Can you work these out from the model? Positions are in its coordinate system, mm. A direction names the side the tool comes from. Give positions to 0.01 mm unless a question says otherwise; leave off trailing zeros. Write each loop counter-clockwise with the first axis right and the second up, starting at its lowest first coordinate (ties: lowest second). Pieces come first, ordered by that corner, then holes. Notation, with made-up numbers: (-18.5, 3) -> (5.5, 3) arc R18 cw to (5.5, 23) -> close; hole circle Ø3 at (67, 88). An arc over 180 degrees is marked (long way). One line per item, written item: value.
from build123d import *

# Parameters (mm, degrees)
SKETCH1_W           = 40
SKETCH1_H           = 27
BOSS_EXTRUDE1_DEPTH = 30
CUT_EXTRUDE1_DEPTH  = 10
SKETCH3_R           = 2.5
CUT_EXTRUDE2_DEPTH  = 30
CUT_EXTRUDE5_START  = -10.62
CUT_EXTRUDE5_DEPTH  = 9
SKETCH10_W          = 20
SKETCH10_H          = 9
CUT_EXTRUDE7_DEPTH  = 6.8
SKETCH12_W          = 20
SKETCH12_H          = 9
CUT_EXTRUDE10_DEPTH = 6.8
FILLET1_R           = 4
SKETCH15_R          = 4.1
CUT_EXTRUDE12_DEPTH = 4
SKETCH16_R          = 2.5
CUT_EXTRUDE13_DEPTH = 4


with BuildPart() as part:
    # Sketch1 → Boss-Extrude1 (new body)
    with BuildSketch(Plane(origin=(0, 0, 0), x_dir=(1, 0, 0), z_dir=(0, 1, 0))):
        with Locations((-2.846153846, 4.313186813)):
            Rectangle(SKETCH1_W, SKETCH1_H)
    extrude(amount=BOSS_EXTRUDE1_DEPTH)

    # Sketch2 → Cut-Extrude1 (cut)
    with BuildSketch(Plane(origin=(0, 0, -17.813186813), x_dir=(-1, 0, 0), z_dir=(0, 0, -1))):
        Polygon((-8.086431081, 26), (-8.086431081, 4), (-0.206431081, 4), (-0.206431081, 7), (-2.866431081, 7), (-2.866431081, 8.008707537), (-0.253846154, 10.628707537), (5.946153846, 10.628707537), (8.558738773, 8.008707537), (8.558738773, 7), (5.898738773, 7), (5.898738773, 4), (13.778738773, 4), (13.778738773, 26), (5.898738773, 26), (5.898738773, 23), (8.558738773, 23), (8.558738773, 21.991292463), (5.938738773, 19.378707537), (-0.246431081, 19.378707537), (-2.866431081, 21.991292463), (-2.866431081, 23), (-0.206431081, 23), (-0.206431081, 26), align=None)
    extrude(amount=-CUT_EXTRUDE1_DEPTH, mode=Mode.SUBTRACT)

    # Sketch3 → Cut-Extrude2 (cut)
    with BuildSketch(Plane.XZ):
        with Locations(Location((10.423846154, 2.186813187, 0), (0, 0, 270))):
            Circle(SKETCH3_R)
        with Locations(Location((-16.116153846, 2.186813187, 0), (0, 0, 90))):
            Circle(SKETCH3_R)
    extrude(amount=-CUT_EXTRUDE2_DEPTH, mode=Mode.SUBTRACT)

    # Sketch8 → Cut-Extrude5 (cut)
    with BuildSketch(Plane.XZ.offset(CUT_EXTRUDE5_START)):
        with BuildLine():
            Line((3.282417725, 9.186813187), (17.153846154, 9.186813187))
            Line((17.153846154, 9.186813187), (17.153846154, -7.813186813))
            Line((17.153846154, -7.813186813), (10.423846154, -7.813186813))
            ThreePointArc((10.423846154, -7.813186813), (1.204301697, -1.686170159), (3.282417725, 9.186813187))
        make_face()
        with BuildLine():
            Line((-22.846153846, -7.813186813), (-16.116153846, -7.813186813))
            ThreePointArc((-16.116153846, -7.813186813), (-6.896609389, -1.686170159), (-8.974725418, 9.186813187))
            Line((-8.974725418, 9.186813187), (-22.846153846, 9.186813187))
            Line((-22.846153846, 9.186813187), (-22.846153846, -7.813186813))
        make_face()
    extrude(amount=-CUT_EXTRUDE5_DEPTH, mode=Mode.SUBTRACT)

    # Sketch10 → Cut-Extrude7 (cut)
    with BuildSketch(Plane.ZY.offset(-8.086431081)):
        with Locations((-7.813186813, 15.12)):
            Rectangle(SKETCH10_W, SKETCH10_H)
    extrude(amount=CUT_EXTRUDE7_DEPTH, mode=Mode.SUBTRACT)

    # Sketch12 → Cut-Extrude10 (cut)
    with BuildSketch(Plane(origin=(-13.778738773, 0, 0), x_dir=(0, 0, -1), z_dir=(1, 0, 0))):
        with Locations((7.813186813, 15.12)):
            Rectangle(SKETCH12_W, SKETCH12_H)
    extrude(amount=CUT_EXTRUDE10_DEPTH, mode=Mode.SUBTRACT)

    # Fillet1
    fillet1_edges = [part.edges().sort_by_distance(p)[0] for p in [
        (17.153846154, 24.81, 9.186813187),
        (-22.846153846, 24.81, 9.186813187),
        (17.153846154, 5.31, 9.186813187),
        (-22.846153846, 5.31, 9.186813187),
    ]]
    fillet(fillet1_edges, radius=FILLET1_R)

    # Sketch15 → Cut-Extrude12 (cut)
    with BuildSketch(Plane(origin=(0, 30, 0), x_dir=(1, 0, 0), z_dir=(0, 1, 0))):
        with Locations(Location((-16.116153846, -2.186813187, 0), (0, 0, 270))):
            Circle(SKETCH15_R)
        with Locations(Location((10.423846154, -2.186813187, 0), (0, 0, 90))):
            Circle(SKETCH15_R)
    extrude(amount=-CUT_EXTRUDE12_DEPTH, mode=Mode.SUBTRACT)

    # Sketch16 → Cut-Extrude13 (cut)
    # profile 1 of 2: a face of its own
    with BuildSketch(Plane.XZ):
        Polygon((-13.749017742, -1.913186813), (-11.381881639, 2.186813187), (-13.749017742, 6.286813187), (-18.48328995, 6.286813187), (-20.850426054, 2.186813187), (-18.48328995, -1.913186813), align=None)
        with Locations(Location((-16.116153846, 2.186813187, 0), (0, 0, 270))):
            Circle(SKETCH16_R, mode=Mode.SUBTRACT)
    # profile 2 of 2: a face of its own
    with BuildSketch(Plane.XZ):
        Polygon((12.790982258, -1.913186813), (15.158118361, 2.186813187), (12.790982258, 6.286813187), (8.05671005, 6.286813187), (5.689573946, 2.186813187), (8.05671005, -1.913186813), align=None)
        with Locations(Location((10.423846154, 2.186813187, 0), (0, 0, 270))):
            Circle(SKETCH16_R, mode=Mode.SUBTRACT)
    extrude(amount=-CUT_EXTRUDE13_DEPTH, mode=Mode.SUBTRACT)


solid = part.part
1) If we section it at B-B (x = 4.5): Write out the boundary of the cut face in (y, z).
Answer list:
outline: (0, -17.81) -> (4, -17.81) -> (4, -7.81) -> (10.62, -7.81) -> (10.62, 9.19) -> (0, 9.19) -> close; (19.62, -7.81) -> (26, -7.81) -> (26, -17.81) -> (30, -17.81) -> (30, 9.19) -> (19.62, 9.19) -> close
2) If we section it at D-D (z = -12.75): Write out the boundary of the cut face in (x, y), and give its area (3 significant figures).
Answer list:
outline: (-22.85, 0) -> (17.15, 0) -> (17.15, 30) -> (-22.85, 30) -> close; hole (-13.78, 4) -> (-5.9, 4) -> (-5.9, 7) -> (-8.56, 7) -> (-8.56, 8.01) -> (-5.95, 10.63) -> (0.25, 10.63) -> (2.87, 8.01) -> (2.87, 7) -> (0.21, 7) -> (0.21, 4) -> (8.09, 4) -> (8.09, 26) -> (0.21, 26) -> (0.21, 23) -> (2.87, 23) -> (2.87, 21.99) -> (0.25, 19.38) -> (-5.94, 19.38) -> (-8.56, 21.99) -> (-8.56, 23) -> (-5.9, 23) -> (-5.9, 26) -> (-13.78, 26) -> close
area: 825 mm^2
3) Will these pins go through, and if not, where does the flat tip stop? pin 1 (4 mm diameter, centred on x = -15, z = 4, fed in from -Y); pin 2 (3.5 mm diameter, centred on x = 12.5, y = 13.5, fed in from +Z).
Answer list:
pin 1: stops at y = 4
pin 2: stops at z = -7.81
4) We'd pull the mould along X, two halves only. Please class faces 1 (the face through (4, 26, -13)), 2 (the face through (-21.71, 24.88, 7.98)), 3 (the face through (17.154, 15, -9)), 4 (the face through (-19.683, 1.972, 0.166)): released by +X, released by -X, zero draft, split by the parting line, or undercut.
Answer list:
face 1: undercut
face 2: released by -X
face 3: released by +X
face 4: undercut
5) If we section it at C-C (y = 12): Write out the boundary of the cut face in (x, z).
Answer list:
outline: (-22.85, -17.81) -> (-13.78, -17.81) -> (-13.78, -7.54) arc R10 cw to (-16.12, -7.81) -> (-22.85, -7.81) -> close; (-8.97, 9.19) arc R10 cw to (-6.98, -1.88) -> (-6.98, -7.81) -> (1.29, -7.81) -> (1.29, -1.88) arc R10 cw to (3.28, 9.19) -> close; (8.09, -17.81) -> (17.15, -17.81) -> (17.15, -7.81) -> (10.42, -7.81) arc R10 cw to (8.09, -7.54) -> close
6) If we section it at A-A (y = 5.75): Write out the boundary of the cut face in (x, z), and give its area (3 significant figures).
Answer list:
outline: (-22.85, -17.81) -> (-13.78, -17.81) -> (-13.78, -7.81) -> (-5.9, -7.81) -> (-5.9, -17.81) -> (0.21, -17.81) -> (0.21, -7.81) -> (8.09, -7.81) -> (8.09, -17.81) -> (17.15, -17.81) -> (17.15, 5.19) arc R4 ccw to (13.15, 9.19) -> (-18.85, 9.19) arc R4 ccw to (-22.85, 5.19) -> close; hole circle Ø5 at (-16.12, 2.19); hole circle Ø5 at (10.42, 2.19)
area: 876 mm^2
7) For faces 5 (the face through (-20.12, 28.03, 1.3)), 6 (the face through (8.206, 7.264, 1.033)), 7 (the face through (6.857, 1.972, 0.166)), 8 (the face through (-5.899, 25, -13)), which set-ups out of +Z, -Z, +X, -X, +Y, -Y let a thin tool reach every point of the face, with its end or its side?
Answer list:
face 5: +Y
face 6: +Y, -Y
face 7: -Y
face 8: -Z
8) I need wall thicknesses on L1, parallel to X at y = 22, z = 2; L2, parallel to Z at x = -16, y = 28.5; L3, parallel to X at y = 10.75, z = -12.5. Which ranges of each line are inside material? Lowest first, please.
Answer list:
L1: x = -22.85 to -18.61, -13.62 to 7.93, 12.92 to 17.15
L2: z = -17.81 to -1.91, 6.29 to 9.19
L3: x = -22.85 to -13.78, 8.09 to 17.15
